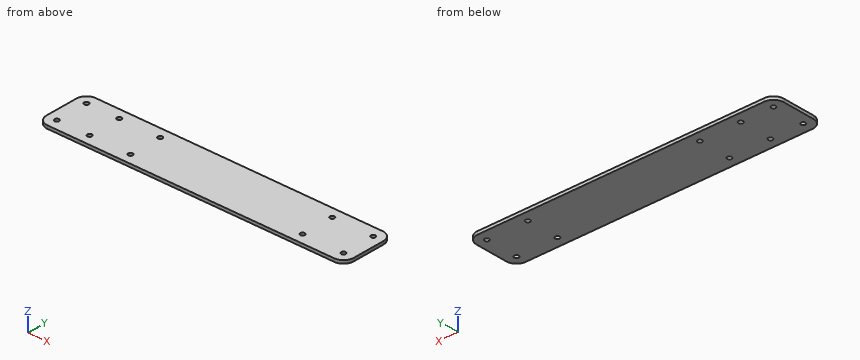
from build123d import *

# Parameters (mm, degrees)
F1_DEPTH = 3
F3_D     = 4.4


with BuildPart() as f1:
    # F0 (on Top) → F1 (new body)
    with BuildSketch(Plane.XY):
        with BuildLine():
            Line((-140, -26), (140, -26))
            ThreePointArc((140, -26), (147.0710678119, -23.0710678119), (150, -16))
            Line((150, -16), (150, 16))
            ThreePointArc((150, 16), (147.0710678119, 23.0710678119), (140, 26))
            Line((140, 26), (-140, 26))
            ThreePointArc((-140, 26), (-147.0710678119, 23.0710678119), (-150, 16))
            Line((-150, 16), (-150, -16))
            ThreePointArc((-150, -16), (-147.0710678119, -23.0710678119), (-140, -26))
        make_face()
    extrude(amount=F1_DEPTH)

    # F3 (through all)
    with Locations(Plane.XY.offset(3)):
        with Locations((-140, 16), (-140, -16), (-108, -16), (-108, 16), (-68, 16), (-68, -16), (140, 16), (100, 16), (100, -16), (140, -16)):
            Hole(F3_D / 2)


solid = f1.part
Source: CAD feature listing. Evaluate the final solid. Frame: model axes, mm. Coordinates: 2 decimals unless noted, no trailing zeros. Answer in a Markdown table with one row per item.
Q1. Ray query, probe 1 along Y at (x, z) = (-68, 0.75); probe 2 along Y at (x, z) = (-108.5, 2); probe 3 along X at (y, z) = (17, 0.8). Return the intervals inside material, ascending. Write a range as from..to.
Answers below:
| item | result |
|---|---|
| probe 1 | y = -26..-18.2, -13.8..13.8, 18.2..26 |
| probe 2 | y = -26..-18.14, -13.86..13.86, 18.14..26 |
| probe 3 | x = -149.95..-141.96, -138.04..-109.96, -106.04..-69.96, -66.04..98.04, 101.96..138.04, 141.96..149.95 |
Q2. First-contact query: pin 1 (7 mm diameter, centred on x = 100, y = 16, fed in from +Z); pin 2 (1 mm diameter, centred on y = 18.5, z = 0.5, fed in from -X). Flat tips, straight axial feed; report the tip coordinate or a pass-through.
Answers below:
| item | result |
|---|---|
| pin 1 | stops at z = 3 |
| pin 2 | stops at x = -149.8 |
Q3. Section A-A on z = 1.2. State how many separate pieces and enclosed holes the cut face has, plus the area to 3 significant figures.
Answers below:
| item | result |
|---|---|
| separate pieces | 1 |
| enclosed holes | 10 |
| area | 15,400 mm^2 |
